Verification items for the finished model (mm, model axes). Face numbers are marked on the shaded views. A direction names the side the tool comes from. Give positions to 0.01 mm unless a question says otherwise; leave off trailing zeros. Order: outer loops, then holes, each group sorted by start corner. A loop starts at its lowest first (then second) coordinate and runs counter-clockwise, first axis right, second up.
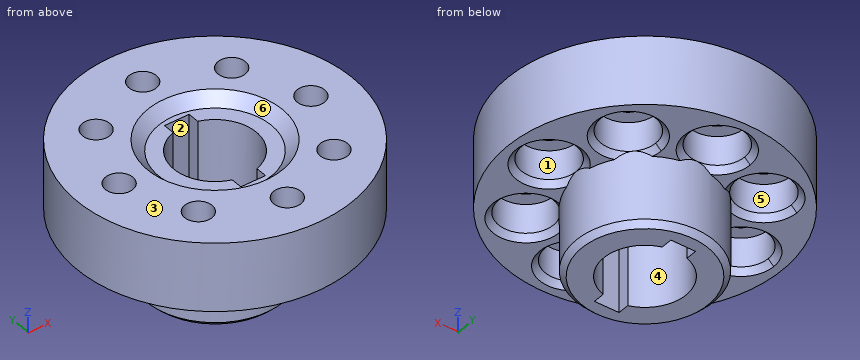
from build123d import *

# Parameters (mm, degrees)
SKETCH1_R                                = 50
BOSS_EXTRUDE1_DEPTH                      = 25
CBORE_FOR_M10_HEX_HEAD_BOLT1_D           = 10
CBORE_FOR_M10_HEX_HEAD_BOLT1_CBORE_D     = 20
CBORE_FOR_M10_HEX_HEAD_BOLT1_CBORE_DEPTH = 12.5
SKETCH5_R                                = 25
BOSS_EXTRUDE2_DEPTH                      = 25
CHAMFER1_SIZE                            = 2
CUT_EXTRUDE1_DEPTH                       = 87.602540436
SKETCH9_R                                = 24.5
CUT_EXTRUDE2_DEPTH                       = 4
CHAMFER2_SIZE                            = 4
CHAMFER3_SIZE                            = 2


# Some blends are built 0.0001 mm under size
with BuildPart() as part:
    # Sketch1 → Boss-Extrude1 (new body)
    with BuildSketch(Plane.XY):
        Circle(SKETCH1_R)
    extrude(amount=-BOSS_EXTRUDE1_DEPTH)

    # CBORE for M10 Hex Head Bolt1 (through all)
    with Locations(Plane(origin=(0, 0, -25), x_dir=(-1, 0, 0), z_dir=(0, 0, -1))):
        with Locations((-24.748737342, 24.748737342), (0, 35), (24.748737342, 24.748737342), (35, 0), (24.748737342, -24.748737342), (0, -35), (-24.748737342, -24.748737342), (-35, 0)):
            CounterBoreHole(CBORE_FOR_M10_HEX_HEAD_BOLT1_D / 2, CBORE_FOR_M10_HEX_HEAD_BOLT1_CBORE_D / 2, CBORE_FOR_M10_HEX_HEAD_BOLT1_CBORE_DEPTH)

    # Sketch5 → Boss-Extrude2 (add)
    with BuildSketch(Plane(origin=(0, 0, -25), x_dir=(-1, 0, 0), z_dir=(0, 0, -1))):
        with Locations(Location((0, 0, 0), (0, 0, 180))):
            Circle(SKETCH5_R)
    extrude(amount=BOSS_EXTRUDE2_DEPTH)

    # Chamfer1
    # the kernel refuses this chamfer: 2 mm, written as the material it takes off along each edge
    with BuildSketch(Plane(origin=(24.748737342, 24.748737342, -25), x_dir=(-1, 0, 0), z_dir=(0, -1, 0))) as chamfer1_piece_1_section:
        Polygon((10 + CHAMFER1_SIZE, 0), (10, -CHAMFER1_SIZE), (10, 0), align=None)
    chamfer1_piece_1 = revolve(axis=Axis((24.748737342, 24.748737342, -25), (0, 0, -1)), revolution_arc=315.000000416, mode=Mode.PRIVATE)
    chamfer1_piece_1 = chamfer1_piece_1 - Plane(origin=(0, 0, -24.034020629), x_dir=(1, 0, 0), z_dir=(0, 0, 1)) * Cylinder(25, 48, mode=Mode.PRIVATE)
    add(chamfer1_piece_1, mode=Mode.SUBTRACT)
    with BuildSketch(Plane(origin=(35, 0, -25), x_dir=(-1, 0, 0), z_dir=(0, -1, 0))) as chamfer1_piece_2_section:
        Polygon((10 + CHAMFER1_SIZE, 0), (10, -CHAMFER1_SIZE), (10, 0), align=None)
    chamfer1_piece_2 = revolve(axis=Axis((35, 0, -25), (0, 0, -1)), mode=Mode.PRIVATE)
    chamfer1_piece_2 = chamfer1_piece_2 - Plane(origin=(0, 0, -24.035090303), x_dir=(1, 0, 0), z_dir=(0, 0, 1)) * Cylinder(25, 48, mode=Mode.PRIVATE)
    add(chamfer1_piece_2, mode=Mode.SUBTRACT)
    with BuildSketch(Plane(origin=(24.748737342, -24.748737342, -25), x_dir=(-1, 0, 0), z_dir=(0, -1, 0))) as chamfer1_piece_3_section:
        Polygon((10 + CHAMFER1_SIZE, 0), (10, -CHAMFER1_SIZE), (10, 0), align=None)
    chamfer1_piece_3 = revolve(axis=Axis((24.748737342, -24.748737342, -25), (0, 0, -1)), revolution_arc=44.999998935, mode=Mode.PRIVATE)
    chamfer1_piece_3 = chamfer1_piece_3 - Plane(origin=(0, 0, -24.295051561), x_dir=(1, 0, 0), z_dir=(0, 0, 1)) * Cylinder(25, 48, mode=Mode.PRIVATE)
    add(chamfer1_piece_3, mode=Mode.SUBTRACT)
    with BuildSketch(Plane(origin=(0, -35, -25), x_dir=(-1, 0, 0), z_dir=(0, -1, 0))) as chamfer1_piece_4_section:
        Polygon((10 + CHAMFER1_SIZE, 0), (10, -CHAMFER1_SIZE), (10, 0), align=None)
    chamfer1_piece_4 = revolve(axis=Axis((0, -35, -25), (0, 0, -1)), revolution_arc=90.00000015, mode=Mode.PRIVATE)
    chamfer1_piece_4 = chamfer1_piece_4 - Plane(origin=(0, 0, -24.021368021), x_dir=(1, 0, 0), z_dir=(0, 0, 1)) * Cylinder(25, 48, mode=Mode.PRIVATE)
    add(chamfer1_piece_4, mode=Mode.SUBTRACT)
    with BuildSketch(Plane(origin=(-24.748737342, -24.748737342, -25), x_dir=(0.7071067835812739, 0.7071067787918212, 0), z_dir=(-0.7071067787918212, 0.7071067835812739, 0))) as chamfer1_piece_5_section:
        Polygon((10 + CHAMFER1_SIZE, 0), (10, -CHAMFER1_SIZE), (10, 0), align=None)
    chamfer1_piece_5 = revolve(axis=Axis((-24.748737342, -24.748737342, -25), (0, 0, -1)), revolution_arc=224.999999806, mode=Mode.PRIVATE)
    chamfer1_piece_5 = chamfer1_piece_5 - Plane(origin=(0, 0, -24.030194299), x_dir=(1, 0, 0), z_dir=(0, 0, 1)) * Cylinder(25, 49, mode=Mode.PRIVATE)
    add(chamfer1_piece_5, mode=Mode.SUBTRACT)
    with BuildSketch(Plane(origin=(-35, 0, -25), x_dir=(-1, 0, 0), z_dir=(0, -1, 0))) as chamfer1_piece_6_section:
        Polygon((10 + CHAMFER1_SIZE, 0), (10, -CHAMFER1_SIZE), (10, 0), align=None)
    chamfer1_piece_6 = revolve(axis=Axis((-35, 0, -25), (0, 0, -1)), revolution_arc=180.000000155, mode=Mode.PRIVATE)
    chamfer1_piece_6 = chamfer1_piece_6 - Plane(origin=(0, 0, -24.027851375), x_dir=(1, 0, 0), z_dir=(0, 0, 1)) * Cylinder(25, 48, mode=Mode.PRIVATE)
    add(chamfer1_piece_6, mode=Mode.SUBTRACT)
    with BuildSketch(Plane(origin=(-24.748737342, 24.748737342, -25), x_dir=(-1, 0, 0), z_dir=(0, -1, 0))) as chamfer1_piece_7_section:
        Polygon((10 + CHAMFER1_SIZE, 0), (10, -CHAMFER1_SIZE), (10, 0), align=None)
    chamfer1_piece_7 = revolve(axis=Axis((-24.748737342, 24.748737342, -25), (0, 0, -1)), revolution_arc=225.000000551, mode=Mode.PRIVATE)
    chamfer1_piece_7 = chamfer1_piece_7 - Plane(origin=(0, 0, -24.030194347), x_dir=(1, 0, 0), z_dir=(0, 0, 1)) * Cylinder(25, 48, mode=Mode.PRIVATE)
    add(chamfer1_piece_7, mode=Mode.SUBTRACT)
    with BuildSketch(Plane(origin=(0, 35, -25), x_dir=(-1, 0, 0), z_dir=(0, -1, 0))) as chamfer1_piece_8_section:
        Polygon((10 + CHAMFER1_SIZE, 0), (10, -CHAMFER1_SIZE), (10, 0), align=None)
    chamfer1_piece_8 = revolve(axis=Axis((0, 35, -25), (0, 0, -1)), revolution_arc=269.999999979, mode=Mode.PRIVATE)
    chamfer1_piece_8 = chamfer1_piece_8 - Plane(origin=(0, 0, -24.032221046), x_dir=(1, 0, 0), z_dir=(0, 0, 1)) * Cylinder(25, 48, mode=Mode.PRIVATE)
    add(chamfer1_piece_8, mode=Mode.SUBTRACT)
    with BuildSketch(Plane(origin=(0, 35, -25), x_dir=(3.7419774552245994e-10, -1.0, 0), z_dir=(1.0, 3.7419774552245994e-10, 0))) as chamfer1_piece_9_section:
        Polygon((10 + CHAMFER1_SIZE, 0), (10, -CHAMFER1_SIZE), (10, 0), align=None)
    chamfer1_piece_9 = revolve(axis=Axis((0, 35, -25), (0, 0, -1)), revolution_arc=90.000000021, mode=Mode.PRIVATE)
    chamfer1_piece_9 = chamfer1_piece_9 - Plane(origin=(0, 0, -24.021368016), x_dir=(1, 0, 0), z_dir=(0, 0, 1)) * Cylinder(25, 48, mode=Mode.PRIVATE)
    add(chamfer1_piece_9, mode=Mode.SUBTRACT)
    with BuildSketch(Plane(origin=(-24.748737342, 24.748737342, -25), x_dir=(0.7071067743839492, -0.7071067879891458, 0), z_dir=(0.7071067879891458, 0.7071067743839492, 0))) as chamfer1_piece_10_section:
        Polygon((10 + CHAMFER1_SIZE, 0), (10, -CHAMFER1_SIZE), (10, 0), align=None)
    chamfer1_piece_10 = revolve(axis=Axis((-24.748737342, 24.748737342, -25), (0, 0, -1)), revolution_arc=134.999999449, mode=Mode.PRIVATE)
    chamfer1_piece_10 = chamfer1_piece_10 - Plane(origin=(0, 0, -24.025029467), x_dir=(1, 0, 0), z_dir=(0, 0, 1)) * Cylinder(25, 48, mode=Mode.PRIVATE)
    add(chamfer1_piece_10, mode=Mode.SUBTRACT)
    with BuildSketch(Plane(origin=(-35, 0, -25), x_dir=(1.0, -2.710294976997066e-09, 0), z_dir=(2.710294976997066e-09, 1.0, 0))) as chamfer1_piece_11_section:
        Polygon((10 + CHAMFER1_SIZE, 0), (10, -CHAMFER1_SIZE), (10, 0), align=None)
    chamfer1_piece_11 = revolve(axis=Axis((-35, 0, -25), (0, 0, -1)), revolution_arc=179.999999845, mode=Mode.PRIVATE)
    chamfer1_piece_11 = chamfer1_piece_11 - Plane(origin=(0, 0, -24.027851322), x_dir=(1, 0, 0), z_dir=(0, 0, 1)) * Cylinder(25, 48, mode=Mode.PRIVATE)
    add(chamfer1_piece_11, mode=Mode.SUBTRACT)
    with BuildSketch(Plane(origin=(-24.748737342, -24.748737342, -25), x_dir=(-1, 0, 0), z_dir=(0, -1, 0))) as chamfer1_piece_12_section:
        Polygon((10 + CHAMFER1_SIZE, 0), (10, -CHAMFER1_SIZE), (10, 0), align=None)
    chamfer1_piece_12 = revolve(axis=Axis((-24.748737342, -24.748737342, -25), (0, 0, -1)), revolution_arc=135.000000194, mode=Mode.PRIVATE)
    chamfer1_piece_12 = chamfer1_piece_12 - Plane(origin=(0, 0, -24.025029447), x_dir=(1, 0, 0), z_dir=(0, 0, 1)) * Cylinder(25, 48, mode=Mode.PRIVATE)
    add(chamfer1_piece_12, mode=Mode.SUBTRACT)
    with BuildSketch(Plane(origin=(0, -35, -25), x_dir=(2.620144484540633e-09, 1.0, 0), z_dir=(-1.0, 2.620144484540633e-09, 0))) as chamfer1_piece_13_section:
        Polygon((10 + CHAMFER1_SIZE, 0), (10, -CHAMFER1_SIZE), (10, 0), align=None)
    chamfer1_piece_13 = revolve(axis=Axis((0, -35, -25), (0, 0, -1)), revolution_arc=269.99999985, mode=Mode.PRIVATE)
    chamfer1_piece_13 = chamfer1_piece_13 - Plane(origin=(0, 0, -24.032221078), x_dir=(1, 0, 0), z_dir=(0, 0, 1)) * Cylinder(25, 48, mode=Mode.PRIVATE)
    add(chamfer1_piece_13, mode=Mode.SUBTRACT)
    with BuildSketch(Plane(origin=(24.748737342, -24.748737342, -25), x_dir=(-0.707106794329391, 0.7071067680437038, 0), z_dir=(-0.7071067680437038, -0.707106794329391, 0))) as chamfer1_piece_14_section:
        Polygon((10 + CHAMFER1_SIZE, 0), (10, -CHAMFER1_SIZE), (10, 0), align=None)
    chamfer1_piece_14 = revolve(axis=Axis((24.748737342, -24.748737342, -25), (0, 0, -1)), revolution_arc=315.000001065, mode=Mode.PRIVATE)
    chamfer1_piece_14 = chamfer1_piece_14 - Plane(origin=(0, 0, -24.034020657), x_dir=(1, 0, 0), z_dir=(0, 0, 1)) * Cylinder(25, 49, mode=Mode.PRIVATE)
    add(chamfer1_piece_14, mode=Mode.SUBTRACT)
    with BuildSketch(Plane(origin=(24.748737342, 24.748737342, -25), x_dir=(-0.7071067863158467, -0.7071067760572484, 0), z_dir=(0.7071067760572484, -0.7071067863158467, 0))) as chamfer1_piece_15_section:
        Polygon((10 + CHAMFER1_SIZE, 0), (10, -CHAMFER1_SIZE), (10, 0), align=None)
    chamfer1_piece_15 = revolve(axis=Axis((24.748737342, 24.748737342, -25), (0, 0, -1)), revolution_arc=44.999999584, mode=Mode.PRIVATE)
    chamfer1_piece_15 = chamfer1_piece_15 - Plane(origin=(0, 0, -24.295051641), x_dir=(1, 0, 0), z_dir=(0, 0, 1)) * Cylinder(25, 48, mode=Mode.PRIVATE)
    add(chamfer1_piece_15, mode=Mode.SUBTRACT)

    # Sketch8 → Cut-Extrude1 (cut, through all)
    with BuildSketch(Plane.XY):
        with BuildLine():
            Line((-4.5, 14.309088021), (-4.5, 18.5))
            Line((-4.5, 18.5), (4.5, 18.5))
            Line((4.5, 18.5), (4.5, 14.309088021))
            ThreePointArc((4.5, 14.309088021), (15, 0), (4.5, -14.309088021))
            Line((4.5, -14.309088021), (4.5, -18.5))
            Line((4.5, -18.5), (-4.5, -18.5))
            Line((-4.5, -18.5), (-4.5, -14.309088021))
            ThreePointArc((-4.5, -14.309088021), (-15, 0), (-4.5, 14.309088021))
        make_face()
    extrude(amount=-CUT_EXTRUDE1_DEPTH, mode=Mode.SUBTRACT)

    # Sketch9 → Cut-Extrude2 (cut)
    with BuildSketch(Plane.XY):
        Circle(SKETCH9_R)
    extrude(amount=-CUT_EXTRUDE2_DEPTH, mode=Mode.SUBTRACT)

    # Chamfer2
    chamfer2_edges = [part.edges().sort_by_distance(p)[0] for p in [
        (-24.5, 0, -4),
    ]]
    chamfer(chamfer2_edges, length=CHAMFER2_SIZE - 0.0001)  # a hair under: the kernel refuses the full size

    # Chamfer3
    chamfer3_edges = [part.edges().sort_by_distance(p)[0] for p in [
        (-25, 0, -50),
    ]]
    chamfer(chamfer3_edges, length=CHAMFER3_SIZE)


solid = part.part
(1) Scan lines: line 1 (Y direction, x = 0, z = -15); line 2 (Y direction, x = -2, z = -10); line 3 (X direction, y = 4, z = -6.5). Record each from-to range of solid material in increasing order.
Solved:
line 1: y = -50 to -45, -25 to -18.5, 18.5 to 25, 45 to 50
line 2: y = -49.96 to -39.58, -30.42 to -18.5, 18.5 to 30.42, 39.58 to 49.96
line 3: x = -49.84 to -38, -32 to -14.46, 14.46 to 32, 38 to 49.84
(2) Release check for a two-part mould opening along Y. For the marked faces 1, 2 and 3 record: pulls with the +Y half, pulls with the -Y half, needs draft (parallel to the pull), parting line crosses it, or undercut.
Solved:
face 1: undercut
face 2: undercut
face 3: needs draft
(3) Set-up check for the marked faces 4, 5 and 6: record each of +Z, -Z, +X, -X, +Y, -Y from which the full face is reachable in a straight line by a thin tool's end or side.
Solved:
face 4: +Z, -Z
face 5: -Z
face 6: +Z
(4) Go/stop test with flat-tipped pins: pin 1 (1 mm diameter, centred on x = 15, z = -34.5, fed in from -Y); pin 2 (8 mm diameter, centred on x = 9.5, y = 11, fed in from -Z); pin 3 (10 mm diameter, centred on x = 1.5, y = -39, fed in from -Z); pin 4 (5 mm diameter, centred on x = -6.5, z = -26, fed in from -Y). Record where each tip stops, or that it passes through.
Solved:
pin 1: stops at y = -20.37
pin 2: stops at z = -50
pin 3: stops at z = -12.5
pin 4: stops at y = -49.82
(5) Section check A-A, the plane z = -40.5. Enter the section's corners in (x, y).
Solved:
outline: circle Ø50 at (0, 0); hole (-4.5, -18.5) - (4.5, -18.5) - (4.5, -14.31) arc R15 ccw to (4.5, 14.31) - (4.5, 18.5) - (-4.5, 18.5) - (-4.5, 14.31) arc R15 ccw to (-4.5, -14.31) - close
